from build123d import *

# Parameters (mm, degrees)
SKETCH_1_W      = 3.333333333
SKETCH_1_H      = 6
SKETCH_1_W_2    = 3.333333334
EXTRUDE_1_DEPTH = 3


with BuildPart() as part:
    # 草图1 → 凸台-拉伸1 (new body)
    with BuildSketch(Plane.XY):
        Polygon((-17, 19.5), (-17, 13), (-19, 13), (-19, -13), (-17, -13), (-17, -19.5), (-10, -19.5), (-10, -13), (-3.5, -13), (-3.5, -19.5), (3.5, -19.5), (3.5, -13), (10, -13), (10, -19.5), (17, -19.5), (17, -13), (19, -13), (19, 13), (17, 13), (17, 19.5), (10, 19.5), (10, 13), (3.5, 13), (3.5, 19.5), (-3.5, 19.5), (-3.5, 13), (-10, 13), (-10, 19.5), align=None)
        with Locations((12.333333334, 0)):
            Rectangle(SKETCH_1_W, SKETCH_1_H, mode=Mode.SUBTRACT)
        with Locations((-12.333333334, 0)):
            Rectangle(SKETCH_1_W, SKETCH_1_H, mode=Mode.SUBTRACT)
        Rectangle(SKETCH_1_W_2, SKETCH_1_H, mode=Mode.SUBTRACT)
    extrude(amount=EXTRUDE_1_DEPTH)


solid = part.part
CAD build for the part. Positions are in the model's coordinates, mm. A direction names the side the tool comes from. Round coordinates to 2 decimals unless told otherwise and drop trailing zeros. Order: outer loops, then holes, each group sorted by start corner. A loop starts at its lowest first (then second) coordinate and runs counter-clockwise, first axis right, second up. Notation, with made-up numbers: (-4.75, -8) - (15.25, -8) arc R7 ccw to (15.25, 0) - close; hole circle Ø11 at (9, -39). An arc over 180 degrees is marked (long way). Return JSON: item names as keys, results as strings.
(1) Pull direction Y, two halves, no side cores. Call faces 1 (the face through (-18, 13, 1)), 2 (the face through (-18, -13, 1)), 3 (the face through (-19, 0, 1)), 4 (the face through (0, 3, 1)): +Y half, -Y half, draft (parallel to the pull), parting line (faces both ways), or undercut.
Answer key:
{"face 1": "+Y half", "face 2": "-Y half", "face 3": "draft", "face 4": "undercut"}
(2) Tool access for faces 5 (the face through (18, 13, 1)), 6 (the face through (18, -13, 1)), 7 (the face through (-14, 0, 1)), 8 (the face through (-10, -16, 1)): list every direction of +Z, -Z, +X, -X, +Y, -Y with a clear straight run to the whole face (end or side of a thin tool).
Answer key:
{"face 5": "+Z, -Z, +X, +Y", "face 6": "+Z, -Z, +X, -Y", "face 7": "+Z, -Z", "face 8": "+Z, -Z, -Y"}
(3) Cut at C-C (y = -15.5). Give the cut face in (x, z), then the cut area to 3 significant figures.
Answer key:
{"outline": "(-17, 0) - (-10, 0) - (-10, 3) - (-17, 3) - close; (-3.5, 0) - (3.5, 0) - (3.5, 3) - (-3.5, 3) - close; (10, 0) - (17, 0) - (17, 3) - (10, 3) - close", "area": "63.0 mm^2"}
(4) Cut at D-D (z = 1.5). State how many separate pieces and enclosed holes the cut face has, then the cut area to 3 significant figures.
Answer key:
{"separate pieces": "1", "enclosed holes": "3", "area": "1,200 mm^2"}
(5) Wall check: probe 1 along X at (y, z) = (15.5, 2.25); probe 2 along X at (y, z) = (-1.5, 1.4); probe 3 along Y at (x, z) = (-9.5, 1.15). Give the ranges that are in metal, low to high. Write a range as from..to.
Answer key:
{"probe 1": "x = -17..-10, -3.5..3.5, 10..17", "probe 2": "x = -19..-14, -10.67..-1.67, 1.67..10.67, 14..19", "probe 3": "y = -13..13"}
(6) Cut at A-A (y = -1). Give the cut face in (x, z).
Answer key:
{"outline": "(-19, 0) - (-14, 0) - (-14, 3) - (-19, 3) - close; (-10.67, 0) - (-1.67, 0) - (-1.67, 3) - (-10.67, 3) - close; (1.67, 0) - (10.67, 0) - (10.67, 3) - (1.67, 3) - close; (14, 0) - (19, 0) - (19, 3) - (14, 3) - close"}
(7) Cut at B-B (x = -0.5). Give the cut face in (y, z).
Answer key:
{"outline": "(-19.5, 0) - (-3, 0) - (-3, 3) - (-19.5, 3) - close; (3, 0) - (19.5, 0) - (19.5, 3) - (3, 3) - close"}
(8) Pin check, flat tips, straight feed: pin 1 Ø1.5 at (x, z) = (-4.5, 0.5) entering from -Y; pin 2 Ø0.9 at (y, z) = (16.5, 1.5) entering from -X; pin 3 Ø1.5 at (y, z) = (16.5, 2) entering from +X. Stop position of each tip, or through.
Answer key:
{"pin 1": "stops at y = -13", "pin 2": "stops at x = -17", "pin 3": "stops at x = 17"}
